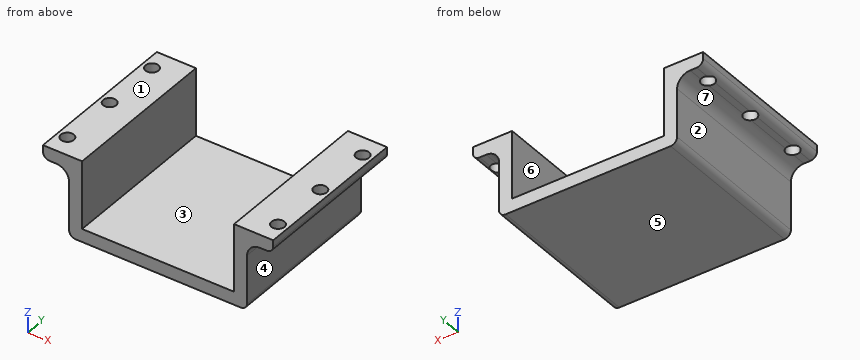
```python
from build123d import *

# Parameters (mm, degrees)
BOSS_EXTRUDE1_DEPTH            = 78
CUT_EXTRUDE1_REACH             = 103.567
SKETCH2_R                      = 3.175
CUT_EXTRUDE1_DIRECTION_2_REACH = 103.567


with BuildPart() as part:
    # Sketch1 → Boss-Extrude1 (new body)
    with BuildSketch(Plane(origin=(0, 0, 0), x_dir=(1, 0, 0), z_dir=(0, 1, 0))):
        with BuildLine():
            Line((-37, -33.02), (-37, 0))
            Line((-37, 0), (37, 0))
            Line((37, 0), (37, -33.02))
            Line((37, -33.02), (56.05, -33.02))
            Line((56.05, -33.02), (56.05, -29.845))
            ThreePointArc((56.05, -29.845), (55.12006403, -27.59993597), (52.875, -26.67))
            Line((52.875, -26.67), (49.7, -26.67))
            ThreePointArc((49.7, -26.67), (45.209871939, -24.810128061), (43.35, -20.32))
            Line((43.35, -20.32), (43.35, 0))
            Line((43.35, 0), (43.35, 3.175))
            ThreePointArc((43.35, 3.175), (42.42006403, 5.42006403), (40.175, 6.35))
            Line((40.175, 6.35), (-40.175, 6.35))
            ThreePointArc((-40.175, 6.35), (-42.42006403, 5.42006403), (-43.35, 3.175))
            Line((-43.35, 3.175), (-43.35, 0))
            Line((-43.35, 0), (-43.35, -20.32))
            ThreePointArc((-43.35, -20.32), (-45.209871939, -24.810128061), (-49.7, -26.67))
            Line((-49.7, -26.67), (-52.875, -26.67))
            ThreePointArc((-52.875, -26.67), (-55.12006403, -27.59993597), (-56.05, -29.845))
            Line((-56.05, -29.845), (-56.05, -33.02))
            Line((-56.05, -33.02), (-37, -33.02))
        make_face()
    extrude(amount=BOSS_EXTRUDE1_DEPTH)

    # Sketch2 → Cut-Extrude1 (cut, up to next)
    with BuildSketch(Plane(origin=(0, 0, 26.67), x_dir=(-1, 0, 0), z_dir=(0, 0, -1)), mode=Mode.PRIVATE) as cut_extrude1_sk1:
        with Locations(Location((-51.2875, 10, 0), (0, 0, 240))):
            Circle(SKETCH2_R)
    cut_extrude1_tool1 = extrude(cut_extrude1_sk1.sketch, amount=-CUT_EXTRUDE1_REACH, mode=Mode.PRIVATE) & part.part
    # Sketch2 → Cut-Extrude1 (cut, up to next)
    with BuildSketch(Plane(origin=(0, 0, 26.67), x_dir=(-1, 0, 0), z_dir=(0, 0, -1)), mode=Mode.PRIVATE) as cut_extrude1_sk2:
        with Locations(Location((-51.2875, 39, 0), (0, 0, 240))):
            Circle(SKETCH2_R)
    cut_extrude1_tool2 = extrude(cut_extrude1_sk2.sketch, amount=-CUT_EXTRUDE1_REACH, mode=Mode.PRIVATE) & part.part
    # Sketch2 → Cut-Extrude1 (cut, up to next)
    with BuildSketch(Plane(origin=(0, 0, 26.67), x_dir=(-1, 0, 0), z_dir=(0, 0, -1)), mode=Mode.PRIVATE) as cut_extrude1_sk3:
        with Locations(Location((-51.2875, 68, 0), (0, 0, 240))):
            Circle(SKETCH2_R)
    cut_extrude1_tool3 = extrude(cut_extrude1_sk3.sketch, amount=-CUT_EXTRUDE1_REACH, mode=Mode.PRIVATE) & part.part
    # Sketch2 → Cut-Extrude1 (cut, up to next)
    with BuildSketch(Plane(origin=(0, 0, 26.67), x_dir=(-1, 0, 0), z_dir=(0, 0, -1)), mode=Mode.PRIVATE) as cut_extrude1_sk4:
        with Locations(Location((51.2875, 68, 0), (0, 0, 180))):
            Circle(SKETCH2_R)
    cut_extrude1_tool4 = extrude(cut_extrude1_sk4.sketch, amount=-CUT_EXTRUDE1_REACH, mode=Mode.PRIVATE) & part.part
    # Sketch2 → Cut-Extrude1 (cut, up to next)
    with BuildSketch(Plane(origin=(0, 0, 26.67), x_dir=(-1, 0, 0), z_dir=(0, 0, -1)), mode=Mode.PRIVATE) as cut_extrude1_sk5:
        with Locations(Location((51.2875, 39, 0), (0, 0, 180))):
            Circle(SKETCH2_R)
    cut_extrude1_tool5 = extrude(cut_extrude1_sk5.sketch, amount=-CUT_EXTRUDE1_REACH, mode=Mode.PRIVATE) & part.part
    # Sketch2 → Cut-Extrude1 (cut, up to next)
    with BuildSketch(Plane(origin=(0, 0, 26.67), x_dir=(-1, 0, 0), z_dir=(0, 0, -1)), mode=Mode.PRIVATE) as cut_extrude1_sk6:
        with Locations(Location((51.2875, 10, 0), (0, 0, 180))):
            Circle(SKETCH2_R)
    cut_extrude1_tool6 = extrude(cut_extrude1_sk6.sketch, amount=-CUT_EXTRUDE1_REACH, mode=Mode.PRIVATE) & part.part
    add(cut_extrude1_tool1.solids().sort_by_distance((51.2875, 10, 26.67))[0], mode=Mode.SUBTRACT)
    add(cut_extrude1_tool2.solids().sort_by_distance((51.2875, 39, 26.67))[0], mode=Mode.SUBTRACT)
    add(cut_extrude1_tool3.solids().sort_by_distance((51.2875, 68, 26.67))[0], mode=Mode.SUBTRACT)
    add(cut_extrude1_tool4.solids().sort_by_distance((-51.2875, 68, 26.67))[0], mode=Mode.SUBTRACT)
    add(cut_extrude1_tool5.solids().sort_by_distance((-51.2875, 39, 26.67))[0], mode=Mode.SUBTRACT)
    add(cut_extrude1_tool6.solids().sort_by_distance((-51.2875, 10, 26.67))[0], mode=Mode.SUBTRACT)

    # Cut-Extrude1 direction 2: up to this face of the body (flat: up to its plane)
    cut_extrude1_direction_2_end = Plane(part.part.faces().sort_by_distance((0, 39, -6.35))[0])
    # Sketch2 → Cut-Extrude1 direction 2 (cut, up to the picked face)
    with BuildSketch(Plane(origin=(0, 0, 26.67), x_dir=(-1, 0, 0), z_dir=(0, 0, -1)), mode=Mode.PRIVATE) as cut_extrude1_direction_2_sk1:
        with Locations(Location((-51.2875, 10, 0), (0, 0, 240))):
            Circle(SKETCH2_R)
    cut_extrude1_direction_2_tool1 = split(extrude(cut_extrude1_direction_2_sk1.sketch, amount=CUT_EXTRUDE1_DIRECTION_2_REACH, mode=Mode.PRIVATE), bisect_by=cut_extrude1_direction_2_end, keep=Keep.BOTH, mode=Mode.PRIVATE)
    # Sketch2 → Cut-Extrude1 direction 2 (cut, up to the picked face)
    with BuildSketch(Plane(origin=(0, 0, 26.67), x_dir=(-1, 0, 0), z_dir=(0, 0, -1)), mode=Mode.PRIVATE) as cut_extrude1_direction_2_sk2:
        with Locations(Location((-51.2875, 39, 0), (0, 0, 240))):
            Circle(SKETCH2_R)
    cut_extrude1_direction_2_tool2 = split(extrude(cut_extrude1_direction_2_sk2.sketch, amount=CUT_EXTRUDE1_DIRECTION_2_REACH, mode=Mode.PRIVATE), bisect_by=cut_extrude1_direction_2_end, keep=Keep.BOTH, mode=Mode.PRIVATE)
    # Sketch2 → Cut-Extrude1 direction 2 (cut, up to the picked face)
    with BuildSketch(Plane(origin=(0, 0, 26.67), x_dir=(-1, 0, 0), z_dir=(0, 0, -1)), mode=Mode.PRIVATE) as cut_extrude1_direction_2_sk3:
        with Locations(Location((-51.2875, 68, 0), (0, 0, 240))):
            Circle(SKETCH2_R)
    cut_extrude1_direction_2_tool3 = split(extrude(cut_extrude1_direction_2_sk3.sketch, amount=CUT_EXTRUDE1_DIRECTION_2_REACH, mode=Mode.PRIVATE), bisect_by=cut_extrude1_direction_2_end, keep=Keep.BOTH, mode=Mode.PRIVATE)
    # Sketch2 → Cut-Extrude1 direction 2 (cut, up to the picked face)
    with BuildSketch(Plane(origin=(0, 0, 26.67), x_dir=(-1, 0, 0), z_dir=(0, 0, -1)), mode=Mode.PRIVATE) as cut_extrude1_direction_2_sk4:
        with Locations(Location((51.2875, 68, 0), (0, 0, 180))):
            Circle(SKETCH2_R)
    cut_extrude1_direction_2_tool4 = split(extrude(cut_extrude1_direction_2_sk4.sketch, amount=CUT_EXTRUDE1_DIRECTION_2_REACH, mode=Mode.PRIVATE), bisect_by=cut_extrude1_direction_2_end, keep=Keep.BOTH, mode=Mode.PRIVATE)
    # Sketch2 → Cut-Extrude1 direction 2 (cut, up to the picked face)
    with BuildSketch(Plane(origin=(0, 0, 26.67), x_dir=(-1, 0, 0), z_dir=(0, 0, -1)), mode=Mode.PRIVATE) as cut_extrude1_direction_2_sk5:
        with Locations(Location((51.2875, 39, 0), (0, 0, 180))):
            Circle(SKETCH2_R)
    cut_extrude1_direction_2_tool5 = split(extrude(cut_extrude1_direction_2_sk5.sketch, amount=CUT_EXTRUDE1_DIRECTION_2_REACH, mode=Mode.PRIVATE), bisect_by=cut_extrude1_direction_2_end, keep=Keep.BOTH, mode=Mode.PRIVATE)
    # Sketch2 → Cut-Extrude1 direction 2 (cut, up to the picked face)
    with BuildSketch(Plane(origin=(0, 0, 26.67), x_dir=(-1, 0, 0), z_dir=(0, 0, -1)), mode=Mode.PRIVATE) as cut_extrude1_direction_2_sk6:
        with Locations(Location((51.2875, 10, 0), (0, 0, 180))):
            Circle(SKETCH2_R)
    cut_extrude1_direction_2_tool6 = split(extrude(cut_extrude1_direction_2_sk6.sketch, amount=CUT_EXTRUDE1_DIRECTION_2_REACH, mode=Mode.PRIVATE), bisect_by=cut_extrude1_direction_2_end, keep=Keep.BOTH, mode=Mode.PRIVATE)
    add(cut_extrude1_direction_2_tool1.solids().sort_by(Axis((51.2875, 10, 26.67), (0, 0, -1)))[0], mode=Mode.SUBTRACT)
    add(cut_extrude1_direction_2_tool2.solids().sort_by(Axis((51.2875, 39, 26.67), (0, 0, -1)))[0], mode=Mode.SUBTRACT)
    add(cut_extrude1_direction_2_tool3.solids().sort_by(Axis((51.2875, 68, 26.67), (0, 0, -1)))[0], mode=Mode.SUBTRACT)
    add(cut_extrude1_direction_2_tool4.solids().sort_by(Axis((-51.2875, 68, 26.67), (0, 0, -1)))[0], mode=Mode.SUBTRACT)
    add(cut_extrude1_direction_2_tool5.solids().sort_by(Axis((-51.2875, 39, 26.67), (0, 0, -1)))[0], mode=Mode.SUBTRACT)
    add(cut_extrude1_direction_2_tool6.solids().sort_by(Axis((-51.2875, 10, 26.67), (0, 0, -1)))[0], mode=Mode.SUBTRACT)


solid = part.part
```
Model file for the job. Use its own axes, mm. Face numbers are marked on the shaded views. A direction names the side the tool comes from. Give positions to 0.01 mm unless a question says otherwise; leave off trailing zeros. Loops run counter-clockwise (first coordinate to the right, second up) from the corner with the lowest first, then second, coordinate; pieces in that order, holes last. Notation, with made-up numbers: (35, -5.75) -> (47, -5.75) arc R13 ccw to (47, -1.75) -> close; hole circle Ø9 at (76.25, 71.5). An arc over 180 degrees is marked (long way). Use CSV: the item, a comma, the result in double quotes. Start each with the question number.
1) Slice it at B-B on y = 62.5. Give the cut face in (x, z) (3 decimals).
2) Flat gauge pins, fed straight in: pin 1 Ø2.5 at (x, y) = (-51, 2.5) entering from -Z; pin 2 Ø3.5 at (x, y) = (-50.5, 53.5) entering from -Z; pin 3 Ø1.5 at (y, z) = (11.5, 16.5) entering from -X. Where does each tip first touch, or does it go through?
3) Mould opens along X. For the marked faces 5, 6 and 7 say: released by +X, released by -X, zero draft, split by the parting line, or undercut.
4) Slice it at D-D on x = 25.5. Give the cut face in (y, z), plus the area to 3 significant figures.
5) Tool access for the marked faces 1, 2, 3 and 4: list every direction of +Z, -Z, +X, -X, +Y, -Y with a clear straight run to the whole face (end or side of a thin tool).
6) Wall check: line 1 (X direction, y = 68, z = 29.75); line 2 (X direction, y = 62.5, z = 5); line 3 (X direction, y = 39, z = 23.5). Give the ranges that are in metal, low to high.
7) Slice it at C-C on y = 10. Give the number of separate pieces and of enclosed holes in the cut face, plus the area to 3 significant figures.
8) Slice it at A-A on z = 19. Give the cut face in (x, y), plus the area to 3 significant figures.
Computed values:
1,outline,"(-56.05, 29.845) arc R3.175 ccw to (-52.875, 26.67) -> (-49.7, 26.67) arc R6.35 cw to (-43.35, 20.32) -> (-43.35, -3.175) arc R3.175 ccw to (-40.175, -6.35) -> (40.175, -6.35) arc R3.175 ccw to (43.35, -3.175) -> (43.35, 20.32) arc R6.35 cw to (49.7, 26.67) -> (52.875, 26.67) arc R3.175 ccw to (56.05, 29.845) -> (56.05, 33.02) -> (37, 33.02) -> (37, 0) -> (-37, 0) -> (-37, 33.02) -> (-56.05, 33.02) -> close"
2,pin 1,"stops at z = 26.67"
2,pin 2,"stops at z = 26.6"
2,pin 3,"stops at x = -43.35"
3,face 5,"zero draft"
3,face 6,"undercut"
3,face 7,"released by -X"
4,outline,"(0, -6.35) -> (78, -6.35) -> (78, 0) -> (0, 0) -> close"
4,area,"495 mm^2"
5,face 1,"+Z, +X, -X, +Y, -Y"
5,face 2,"-Z, -X, +Y, -Y"
5,face 3,"+Z, +Y, -Y"
5,face 4,"-Z, +X, +Y, -Y"
6,line 1,"x = -56.05 to -54.46, -48.11 to -37, 37 to 48.11, 54.46 to 56.05"
6,line 2,"x = -43.35 to -37, 37 to 43.35"
6,line 3,"x = -44.2 to -37, 37 to 44.2"
7,separate pieces,"3"
7,enclosed holes,"0"
7,area,"1,060 mm^2"
8,outline,"(-43.35, 0) -> (-37, 0) -> (-37, 78) -> (-43.35, 78) -> close; (37, 0) -> (43.35, 0) -> (43.35, 78) -> (37, 78) -> close"
8,area,"991 mm^2"
